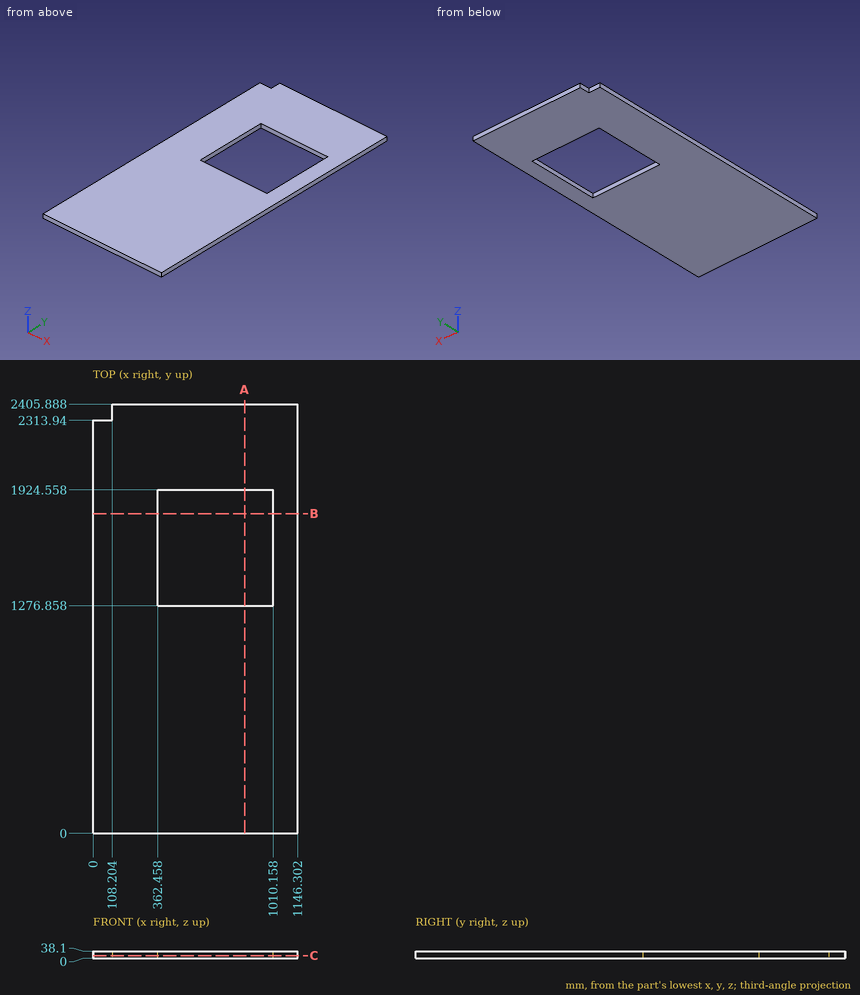
Check sheet for the drawn part. Datum: minimum x, y, z corner. Units: mm. Coordinates: 2 decimals unless noted, no trailing zeros. Loops run counter-clockwise (first coordinate to the right, second up) from the corner with the lowest first, then second, coordinate; pieces in that order, holes last. Notation, with made-up numbers: M 52,14 L 65,14 A16 cw 65,42 Z; hole C 35,70 d7. An arc over 180 degrees is marked long. Answer as a JSON object with one key per item and string values.
1. Depth check by flat-ended pin: P1, Ø11.5, axis at y = 1749, z = 22, coming from the -X side; P2, Ø19, axis at y = 2372.5, z = 25, coming from the -X side. Enter the tip coordinate at first touch or a pass-through.
Outcome:
{"P1": "x = 0", "P2": "x = 108.2"}
2. Sectioned sample at C-C on z = 14. Record the cut outline in (x, y), and give its area (3 significant figures).
Outcome:
{"outline": "M 0,0 L 1146.3,0 L 1146.3,2405.89 L 108.2,2405.89 L 108.2,2313.94 L 0,2313.94 Z; hole M 362.46,1276.86 L 1010.16,1276.86 L 1010.16,1924.56 L 362.46,1924.56 Z", "area": "2,330,000 mm²"}
3. Scan lines: L1, parallel to X at y = 1606, z = 16; L2, parallel to Y at x = 383, z = 32.5; L3, parallel to Y at x = 103, z = 4. Record each from-to range of solid material in increasing order. Write a range as from..to.
Outcome:
{"L1": "0..362.46, 1010.16..1146.3", "L2": "0..1276.86, 1924.56..2405.89", "L3": "0..2313.94"}
4. Sectioned sample at A-A on x = 849. Record the cut outline in (y, z), and give its area (3 significant figures).
Outcome:
{"outline": "M 0,0 L 1276.86,0 L 1276.86,38.1 L 0,38.1 Z; M 1924.56,0 L 2405.89,0 L 2405.89,38.1 L 1924.56,38.1 Z", "area": "67,000 mm²"}
5. Sectioned sample at B-B on y = 1791. Record the cut outline in (x, z), and give its area (3 significant figures).
Outcome:
{"outline": "M 0,0 L 362.46,0 L 362.46,38.1 L 0,38.1 Z; M 1010.16,0 L 1146.3,0 L 1146.3,38.1 L 1010.16,38.1 Z", "area": "19,000 mm²"}
